```python
from build123d import *

# Parameters (mm, degrees)
SKETCH_1_R          = 85
EXTRUDE_1_DEPTH     = 10
SKETCH_2_W          = 260
SKETCH_2_H          = 80
EXTRUDE_2_DEPTH     = 10
SKETCH_3_R          = 85
EXTRUDE_3_DEPTH     = 10
SKETCH_4_R          = 10
SKETCH_4_R_2        = 3.25
SKETCH_4_R_3        = 50
SKETCH_4_R_4        = 2.75
SKETCH_4_R_5        = 2.1
SKETCH_4_R_6        = 5.1
CUT_EXTRUDE_1_DEPTH = 11


with BuildPart() as part:
    # 草图1 → 凸台-拉伸1 (new body)
    with BuildSketch(Plane.XY):
        Circle(SKETCH_1_R)
    extrude(amount=EXTRUDE_1_DEPTH)

    # 草图2 → 凸台-拉伸2 (add)
    with BuildSketch(Plane.XY):
        with Locations((130, 0)):
            Rectangle(SKETCH_2_W, SKETCH_2_H)
    extrude(amount=EXTRUDE_2_DEPTH)

    # 草图3 → 凸台-拉伸3 (add)
    with BuildSketch(Plane.XY):
        with Locations((260, 0)):
            Circle(SKETCH_3_R)
    extrude(amount=EXTRUDE_3_DEPTH)

    # 草图4 → 切除-拉伸1 (cut)
    with BuildSketch(Plane(origin=(0, 0, 0), x_dir=(-1, 0, 0), z_dir=(0, 0, -1))):
        Circle(SKETCH_4_R)
        with Locations((-22, 0)):
            Circle(SKETCH_4_R_2)
        with Locations((-11, 19.052558883)):
            Circle(SKETCH_4_R_2)
        with Locations((11, 19.052558883)):
            Circle(SKETCH_4_R_2)
        with Locations((22, 0)):
            Circle(SKETCH_4_R_2)
        with Locations((11, -19.052558883)):
            Circle(SKETCH_4_R_2)
        with Locations((-11, -19.052558883)):
            Circle(SKETCH_4_R_2)
        with Locations((-260, 0)):
            Circle(SKETCH_4_R_3)
        with Locations((-316, 0)):
            Circle(SKETCH_4_R_4)
        with Locations((-308.497422612, 28)):
            Circle(SKETCH_4_R_4)
        with Locations((-288, 48.497422612)):
            Circle(SKETCH_4_R_4)
        with Locations((-260, 56)):
            Circle(SKETCH_4_R_4)
        with Locations((-232, 48.497422612)):
            Circle(SKETCH_4_R_4)
        with Locations((-211.502577388, 28)):
            Circle(SKETCH_4_R_4)
        with Locations((-204, 0)):
            Circle(SKETCH_4_R_4)
        with Locations((-211.502577388, -28)):
            Circle(SKETCH_4_R_4)
        with Locations((-232, -48.497422612)):
            Circle(SKETCH_4_R_4)
        with Locations((-260, -56)):
            Circle(SKETCH_4_R_4)
        with Locations((-288, -48.497422612)):
            Circle(SKETCH_4_R_4)
        with Locations((-308.497422612, -28)):
            Circle(SKETCH_4_R_4)
        with Locations((-312.622786764, 19.153128026)):
            Circle(SKETCH_4_R_5)
        with Locations((-240.846871974, 52.622786764)):
            Circle(SKETCH_4_R_5)
        with Locations((-207.377213236, -19.153128026)):
            Circle(SKETCH_4_R_5)
        with Locations((-279.153128026, -52.622786764)):
            Circle(SKETCH_4_R_5)
        with Locations((-70, 0)):
            Circle(SKETCH_4_R_6)
        with Locations((-260, -70)):
            Circle(SKETCH_4_R_6)
    extrude(amount=-CUT_EXTRUDE_1_DEPTH, mode=Mode.SUBTRACT)


solid = part.part
```
The model under review builds one solid part; all positions refer to its coordinate system, in mm. A direction names the side the tool comes from. Round coordinates to 2 decimals unless told otherwise and drop trailing zeros. Order: outer loops, then holes, each group sorted by start corner. A loop starts at its lowest first (then second) coordinate and runs counter-clockwise, first axis right, second up. Notation, with made-up numbers: (-26.75, -29) - (0.25, -29) arc R16 ccw to (0.25, -4) - close; hole circle Ø5 at (-25.75, 17). An arc over 180 degrees is marked (long way). Answer in a Markdown table with one row per item.
(1) For line 1 (Y direction, x = 232, z = 6.5); line 2 (X direction, y = -44.5, z = 6.75); line 3 (Y direction, x = 240.5, z = 5), list the stretches that pass through material, from the lowest coordinate up. Write a range as from..to.
Result set:
| item | result |
|---|---|
| line 1 | y = -80.26..-51.25, -45.75..-41.42, 41.42..45.75, 51.25..80.26 |
| line 2 | x = -72.42..72.42, 187.58..237.2, 282.8..332.42 |
| line 3 | y = -82.73..-46.04, 46.04..50.55, 54.69..82.73 |
(2) Take a section at D-D on x = 272. Write out the cut boundary in (y, z), plus the area to 3 significant figures.
Result set:
| item | result |
|---|---|
| outline | (-84.15, 0) - (-48.54, 0) - (-48.54, 10) - (-84.15, 10) - close; (48.54, 0) - (84.15, 0) - (84.15, 10) - (48.54, 10) - close |
| area | 712 mm2 |
(3) Take a section at A-A on x = 70. Write out the cut boundary in (y, z), plus the area to 3 significant figures.
Result set:
| item | result |
|---|---|
| outline | (-48.22, 0) - (-5.1, 0) - (-5.1, 10) - (-48.22, 10) - close; (5.1, 0) - (48.22, 0) - (48.22, 10) - (5.1, 10) - close |
| area | 862 mm2 |
(4) Take a section at C-C on z = 7. Count the separate pieces of the cut face and the enclosed holes in it, plus the area to 3 significant figures.
Result set:
| item | result |
|---|---|
| separate pieces | 1 |
| enclosed holes | 26 |
| area | 44,200 mm2 |
(5) Mouldability with a two-part tool opening along X and no side actions: class faces 4 (the face through (309.95, 2.2, 4.93)), 5 (the face through (127, 1, 10)) as released by +X, released by -X, zero draft, split by the parting line, or undercut.
Result set:
| item | result |
|---|---|
| face 4 | undercut |
| face 5 | zero draft |
(6) Machinability: for faces 1 (the face through (129, -40, 5)), 2 (the face through (129, 40, 5)), 3 (the face through (-84.94, 3.15, 4.93)), which of the approach directions +Z, -Z, +X, -X, +Y, -Y give a long, thin tool a straight path to every point of the face, cutting with its end or side? Answer none if there is none.
Result set:
| item | result |
|---|---|
| face 1 | +Z, -Z, -Y |
| face 2 | +Z, -Z, +Y |
| face 3 | +Z, -Z |
(7) Clearance check with flat-ended pins moving along their axes: P1, Ø3, axis at x = 144.5, z = 6.5, coming from the +Y side; P2, Ø3, axis at x = 143, z = 3, coming from the -Y side; P3, Ø1.5, axis at y = 39, z = 3.5, coming from the -X side. State where each tip first meets the part, or that it passes through.
Result set:
| item | result |
|---|---|
| P1 | stops at y = 40 |
| P2 | stops at y = -40 |
| P3 | stops at x = -75.91 |
(8) Take a section at B-B on y = -70. Write out the cut boundary in (x, z).
Result set:
| item | result |
|---|---|
| outline | (-48.22, 0) - (48.22, 0) - (48.22, 10) - (-48.22, 10) - close; (211.78, 0) - (254.9, 0) - (254.9, 10) - (211.78, 10) - close; (265.1, 0) - (308.22, 0) - (308.22, 10) - (265.1, 10) - close |
